```python
from build123d import *

# Parameters (mm, degrees)
BOSS_EXTRUDE1_DEPTH = 226.1
SKETCH2_R           = 4
SKETCH2_R_2         = 6
CUT_EXTRUDE1_DEPTH  = 230.733454246
SKETCH3_R           = 4
CUT_EXTRUDE2_DEPTH  = 230.733454246


with BuildPart() as part:
    # Sketch1 → Boss-Extrude1 (new, symmetric)
    with BuildSketch(Plane.XY):
        Polygon((0, 2.5), (0, 30), (2.5, 30), (2.5, 2.5), (30, 2.5), (30, 0), (0, 0), align=None)
    extrude(amount=BOSS_EXTRUDE1_DEPTH, both=True)

    # Sketch2 → Cut-Extrude1 (cut, through all)
    with BuildSketch(Plane(origin=(0, 2.5, 0), x_dir=(1, 0, 0), z_dir=(0, 1, 0))):
        with Locations(Location((17.5, 208.6, 0), (0, 0, 180))):
            Circle(SKETCH2_R)
        with Locations(Location((17.5, -213.6, 0), (0, 0, 180))):
            Circle(SKETCH2_R)
        with Locations(Location((15, -100, 0), (0, 0, 180))):
            Circle(SKETCH2_R_2)
        with Locations(Location((15, 100, 0), (0, 0, 180))):
            Circle(SKETCH2_R_2)
        with Locations(Location((15, 0, 0), (0, 0, 180))):
            Circle(SKETCH2_R_2)
    extrude(amount=-CUT_EXTRUDE1_DEPTH, mode=Mode.SUBTRACT)

    # Sketch3 → Cut-Extrude2 (cut, through all)
    with BuildSketch(Plane(origin=(2.5, 0, 0), x_dir=(0, 0, -1), z_dir=(1, 0, 0))):
        with Locations((-213.6, 15)):
            Circle(SKETCH3_R)
        with Locations(Location((213.6, 15, 0), (0, 0, 180))):
            Circle(SKETCH3_R)
    extrude(amount=-CUT_EXTRUDE2_DEPTH, mode=Mode.SUBTRACT)


solid = part.part
```
Verification items for the finished model (mm, model axes). A direction names the side the tool comes from. Give positions to 0.01 mm unless a question says otherwise; leave off trailing zeros. Loops run counter-clockwise (first coordinate to the right, second up) from the corner with the lowest first, then second, coordinate; pieces in that order, holes last.
1. Go/stop test with flat-tipped pins: pin 1 Ø10.5 at (x, z) = (17.5, -208.6) entering from +Y; pin 2 Ø5 at (y, z) = (13.5, -166) entering from +X. Record where each tip stops, or that it passes through.
2. Section check A-A, the plane z = 100. Enter the section's corners in (x, y).
3. Section check B-B, the plane y = 15. Enter the section's corners in (x, z), then the cut area to 3 significant figures.
4. Mould release check, pull along X, two halves, no side actions. Record for faces 1 (the cylindrical face through (18.021, 1.268, -204.634)), 2 (the flat face through (2.5, 16, 3)), 3 (the cylindrical face through (1.268, 13.799, -209.785)): released by +X, released by -X, zero draft, split by the parting line, or undercut.
5. Thickness scan on line 1 (Z direction, x = 15, y = 1.2); line 2 (Y direction, x = 14.5, z = -204.5). Record the ranges inside material, lowest first.
6. Section check C-C, the plane z = 213.6. Enter the section's corners in (x, y).
7. Section check D-D, the plane z = -124. Enter the section's corners in (x, y).
8. Set-up check for faces 4 (the flat face through (22, 2.5, 3)), 5 (the cylindrical face through (15.78, 1.27, -94.05)): record each of +Z, -Z, +X, -X, +Y, -Y from which the full face is reachable in a straight line by a thin tool's end or side.
Geometry says:
1. pin 1: stops at y = 2.5
1. pin 2: stops at x = 2.5
2. outline: (0, 0) - (9, 0) - (9, 2.5) - (2.5, 2.5) - (2.5, 30) - (0, 30) - close; (21, 0) - (30, 0) - (30, 2.5) - (21, 2.5) - close
3. outline: (0, -226.1) - (2.5, -226.1) - (2.5, -217.6) - (0, -217.6) - close; (0, -209.6) - (2.5, -209.6) - (2.5, 209.6) - (0, 209.6) - close; (0, 217.6) - (2.5, 217.6) - (2.5, 226.1) - (0, 226.1) - close
3. area: 1,090 mm2
4. face 1: undercut
4. face 2: released by +X
4. face 3: zero draft
5. line 1: z = -226.1 to -211.72, -205.48 to -106, -94 to -6, 6 to 94, 106 to 210.48, 216.72 to 226.1
5. line 2: y = 0 to 2.5
6. outline: (0, 0) - (13.5, 0) - (13.5, 2.5) - (2.5, 2.5) - (2.5, 11) - (0, 11) - close; (0, 19) - (2.5, 19) - (2.5, 30) - (0, 30) - close; (21.5, 0) - (30, 0) - (30, 2.5) - (21.5, 2.5) - close
7. outline: (0, 0) - (30, 0) - (30, 2.5) - (2.5, 2.5) - (2.5, 30) - (0, 30) - close
8. face 4: +Z, -Z, +X, +Y
8. face 5: +Y, -Y
